Job drawing, mm, ordinate dimensions from the low corner. One solid piece. Coordinates: 2 decimals unless noted, no trailing zeros. Order: outer loops, then holes, each group sorted by start corner. A loop starts at its lowest first (then second) coordinate and runs counter-clockwise, first axis right, second up. Notation, with made-up numbers: (10, -33) - (17, -33) arc R15 ccw to (17, -20) - close; hole circle Ø2 at (5.5, 22). An arc over 180 degrees is marked (long way). Use one line per item in the form item = value.
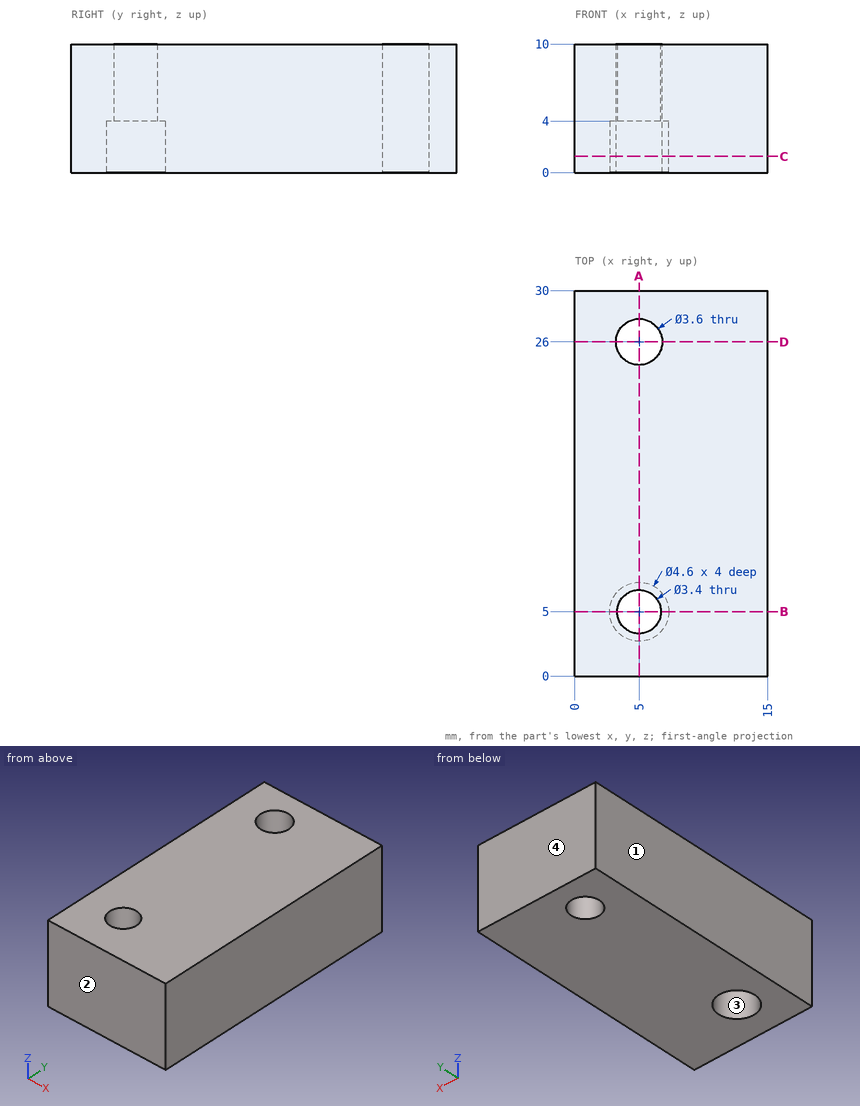
Item 1: Two-plate mould, pull along Y, no slides. Class the marked faces 1, 2, 3 and 4: +Y half, -Y half, draft (parallel to the pull), parting line (faces both ways), or undercut.
Derived:
face_1 = draft
face_2 = -Y half
face_3 = undercut
face_4 = +Y half
Item 2: Cut at C-C, the plane z = 1.25. Write the cut outline in (x, y), plus the area to 3 significant figures.
Derived:
outline = (0, 0) - (15, 0) - (15, 30) - (0, 30) - close; hole circle Ø4.6 at (5, 5); hole circle Ø3.6 at (5, 26)
area = 423 mm²
Item 3: Drop a flat-ended pin along its axis: pin 1 (4 mm diameter, centred on x = 5, y = 5, fed in from -Z). Give the stop position or say it passes through.
Derived:
pin_1 = 4
Item 4: Cut at D-D, the plane y = 26. Write the cut outline in (x, z), plus the area to 3 significant figures.
Derived:
outline = (0, 0) - (3.2, 0) - (3.2, 10) - (0, 10) - close; (6.8, 0) - (15, 0) - (15, 10) - (6.8, 10) - close
area = 114 mm²
Item 5: Cut at B-B, the plane y = 5. Write the cut outline in (x, z), plus the area to 3 significant figures.
Derived:
outline = (0, 0) - (2.7, 0) - (2.7, 4) - (3.3, 4) - (3.3, 10) - (0, 10) - close; (6.7, 4) - (7.3, 4) - (7.3, 0) - (15, 0) - (15, 10) - (6.7, 10) - close
area = 111 mm²
Item 6: Cut at A-A, the plane x = 5. Write the cut outline in (y, z), plus the area to 3 significant figures.
Derived:
outline = (0, 0) - (2.7, 0) - (2.7, 4) - (3.3, 4) - (3.3, 10) - (0, 10) - close; (6.7, 4) - (7.3, 4) - (7.3, 0) - (24.2, 0) - (24.2, 10) - (6.7, 10) - close; (27.8, 0) - (30, 0) - (30, 10) - (27.8, 10) - close
area = 225 mm²
Item 7: Drill centre lines: line 1 (Y direction, x = 5, z = 2.75); line 2 (Y direction, x = 5, z = 7.6); line 3 (X direction, y = 5, z = 1.1). Where is each one in solid material? Low to high. Write a range as [from, to].
Derived:
line_1 = [0, 2.7], [7.3, 24.2], [27.8, 30]
line_2 = [0, 3.3], [6.7, 24.2], [27.8, 30]
line_3 = [0, 2.7], [7.3, 15]
